from build123d import *

# Parameters (mm, degrees)
SKETCH1_R           = 2
SKETCH1_R_2         = 3.125
SKETCH1_R_3         = 1.7
BOSS_EXTRUDE1_DEPTH = 10
FILLET2_R           = 3
FILLET1_R           = 2
SKETCH1_4_R         = 3.125
CUT_EXTRUDE3_DEPTH  = 5.07
SKETCH1_7_R         = 1.7
CUT_EXTRUDE6_DEPTH  = 10
CUT_EXTRUDE5_DEPTH  = 3
SKETCH1_5_R         = 2
CUT_EXTRUDE4_DEPTH  = 2.48
SKETCH4_R           = 1.5
CUT_EXTRUDE7_DEPTH  = 10
SKETCH5_R           = 2.725
CUT_EXTRUDE8_DEPTH  = 2.8


with BuildPart() as part:
    # Sketch1 → Boss-Extrude1 (new body)
    with BuildSketch(Plane(origin=(0, 0, 0), x_dir=(1, 0, 0), z_dir=(0, 1, 0))):
        with BuildLine():
            ThreePointArc((-11.409245094, 8.977987014), (-9.849239736, 9.28), (-8.289234378, 8.977987014))
            ThreePointArc((-8.289234378, 8.977987014), (-5.835653376, 8.254222737), (-3.289234378, 8.01))
            Line((-3.289234378, 8.01), (38.12, 8.01))
            Line((38.12, 8.01), (38.12, -3.81))
            Line((38.12, -3.81), (28.478275237, -3.81))
            Line((28.478275237, -3.81), (26.178275237, 0))
            Line((26.178275237, 0), (-26.178275237, 0))
            Line((-26.178275237, 0), (-28.478275237, -3.81))
            Line((-28.478275237, -3.81), (-38.12, -3.81))
            Line((-38.12, -3.81), (-38.12, 8.01))
            Line((-38.12, 8.01), (-16.409245094, 8.01))
            ThreePointArc((-16.409245094, 8.01), (-13.862826096, 8.254222737), (-11.409245094, 8.977987014))
        make_face()
        with Locations((22, 4.005)):
            Circle(SKETCH1_R, mode=Mode.SUBTRACT)
        with Locations((-22, 4.005)):
            Circle(SKETCH1_R, mode=Mode.SUBTRACT)
        with Locations((-32.12, 1.98)):
            Circle(SKETCH1_R_2, mode=Mode.SUBTRACT)
        with Locations((32.12, 1.98)):
            Circle(SKETCH1_R_2, mode=Mode.SUBTRACT)
        with Locations((-9.849239736, 5.1)):
            Circle(SKETCH1_R_3, mode=Mode.SUBTRACT)
        with BuildLine():
            ThreePointArc((11.912105026, 2.53), (14.127105026, 4.745), (11.912105026, 6.96))
            Line((11.912105026, 6.96), (5.992105026, 6.96))
            ThreePointArc((5.992105026, 6.96), (3.777105026, 4.745), (5.992105026, 2.53))
            Line((5.992105026, 2.53), (11.912105026, 2.53))
        make_face(mode=Mode.SUBTRACT)
        with Locations((-22, 4.005)):
            Circle(SKETCH1_R)
        with Locations((-9.849239736, 5.1)):
            Circle(SKETCH1_R_3)
        with Locations((-32.12, 1.98)):
            Circle(SKETCH1_R_2)
        with BuildLine():
            Line((5.992105026, 2.53), (11.912105026, 2.53))
            ThreePointArc((11.912105026, 2.53), (14.127105026, 4.745), (11.912105026, 6.96))
            Line((11.912105026, 6.96), (5.992105026, 6.96))
            ThreePointArc((5.992105026, 6.96), (3.777105026, 4.745), (5.992105026, 2.53))
        make_face()
        with Locations((22, 4.005)):
            Circle(SKETCH1_R)
        with Locations((32.12, 1.98)):
            Circle(SKETCH1_R_2)
    extrude(amount=-BOSS_EXTRUDE1_DEPTH)

    # Fillet2
    fillet2_edges = [part.edges().sort_by_distance(p)[0] for p in [
        (28.478275237, -5, 3.81),
        (-28.478275237, -5, 3.81),
    ]]
    fillet(fillet2_edges, radius=FILLET2_R)

    # Fillet1
    fillet1_edges = [part.edges().sort_by_distance(p)[0] for p in [
        (26.178275237, -5, 0),
        (-26.178275237, -5, 0),
    ]]
    fillet(fillet1_edges, radius=FILLET1_R)

    # Sketch1_4 → Cut-Extrude3 (cut)
    with BuildSketch(Plane(origin=(0, 0, 0), x_dir=(1, 0, 0), z_dir=(0, 1, 0))):
        with Locations((32.12, 1.98)):
            Circle(SKETCH1_4_R)
        with Locations((-32.12, 1.98)):
            Circle(SKETCH1_4_R)
    extrude(amount=-CUT_EXTRUDE3_DEPTH, mode=Mode.SUBTRACT)

    # Sketch1_7 → Cut-Extrude6 (cut)
    with BuildSketch(Plane(origin=(0, 0, 0), x_dir=(1, 0, 0), z_dir=(0, 1, 0))):
        with Locations((-9.849239736, 5.1)):
            Circle(SKETCH1_7_R)
    extrude(amount=-CUT_EXTRUDE6_DEPTH, mode=Mode.SUBTRACT)

    # Sketch1_6 → Cut-Extrude5 (cut)
    with BuildSketch(Plane(origin=(0, 0, 0), x_dir=(1, 0, 0), z_dir=(0, 1, 0))):
        with BuildLine():
            Line((5.992105026, 2.53), (11.912105026, 2.53))
            ThreePointArc((11.912105026, 2.53), (14.127105026, 4.745), (11.912105026, 6.96))
            Line((11.912105026, 6.96), (5.992105026, 6.96))
            ThreePointArc((5.992105026, 6.96), (3.777105026, 4.745), (5.992105026, 2.53))
        make_face()
    extrude(amount=-CUT_EXTRUDE5_DEPTH, mode=Mode.SUBTRACT)

    # Sketch1_5 → Cut-Extrude4 (cut)
    with BuildSketch(Plane(origin=(0, 0, 0), x_dir=(1, 0, 0), z_dir=(0, 1, 0))):
        with Locations((-22, 4.005)):
            Circle(SKETCH1_5_R)
        with Locations((22, 4.005)):
            Circle(SKETCH1_5_R)
    extrude(amount=-CUT_EXTRUDE4_DEPTH, mode=Mode.SUBTRACT)

    # Sketch4 → Cut-Extrude7 (cut)
    with BuildSketch(Plane(origin=(0, 0, 0), x_dir=(1, 0, 0), z_dir=(0, 1, 0))):
        with Locations((-22, 4.005)):
            Circle(SKETCH4_R)
        with Locations((22, 4.005)):
            Circle(SKETCH4_R)
    extrude(amount=-CUT_EXTRUDE7_DEPTH, mode=Mode.SUBTRACT)

    # Sketch5 → Cut-Extrude8 (cut)
    with BuildSketch(Plane.XZ.offset(10)):
        with Locations((22, -4.005)):
            Circle(SKETCH5_R)
        with Locations((-22, -4.005)):
            Circle(SKETCH5_R)
    extrude(amount=-CUT_EXTRUDE8_DEPTH, mode=Mode.SUBTRACT)


solid = part.part
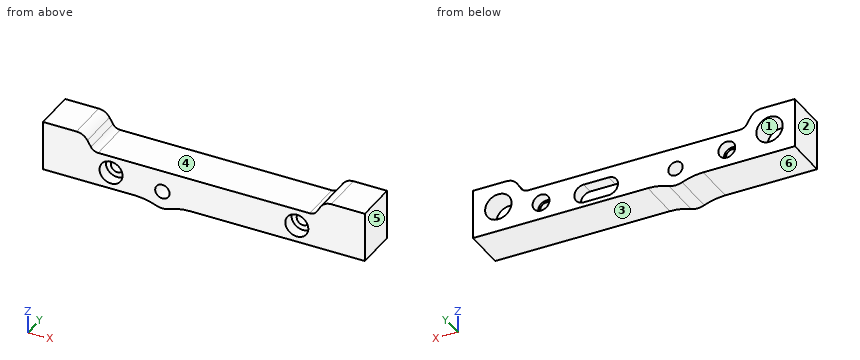
Design review of the part built by this model. Coordinates are the model's own, in mm. Face numbers are marked on the shaded views. A direction names the side the tool comes from. Give positions to 0.01 mm unless a question says otherwise; leave off trailing zeros. Loops run counter-clockwise (first coordinate to the right, second up) from the corner with the lowest first, then second, coordinate; pieces in that order, holes last. Notation, with made-up numbers: (2.5, 66.5) - (41.5, 66.5) arc R12 ccw to (41.5, 81.5) - close; hole circle Ø7 at (-17.5, 59). An arc over 180 degrees is marked (long way). Use CSV: the item, a comma, the result in double quotes. Start each with the question number.
1. Machinability: for the marked faces 1, 2 and 3, which of the approach directions +Z, -Z, +X, -X, +Y, -Y give a long, thin tool a straight path to every point of the face, cutting with its end or side? Answer none if there is none.
2. Wall thickness on L1, parallel to X at y = -2.95, z = -1.98 (3 decimals); L2, parallel to Z at x = 22, y = -4 (3 decimals); L3, parallel to X at y = -2.25, z = -5.5: over which ranges is each line inside the solid? List them lowest first.
3. Add section A-A (x = 22). State the section outline as (y, z) points (3 decimals).
4. Add section B-B (x = -32.12). State the section outline as (y, z) points (3 decimals), plus the area to 3 significant figures.
5. Draft analysis for pull direction X (two halves, no side actions). For the marked faces 4, 5 and 6, state which applies: released by +X, released by -X, zero draft, split by the parting line, or undercut.
6. Add section D-D (y = -0.75). Count the separate pieces of the cut face and the enclosed holes in it, plus the area to 3 significant figures.
7. Insertion check: P1, Ø2.5, axis at x = 8.5, y = -1.5, coming from the +Z side; P2, Ø3.5, axis at x = -22, z = -4.005, coming from the -Y side; P3, Ø3.5, axis at x = 22, z = -4.005, coming from the +Y side. Each pin has a flat end and moves straight along its axis. Give the tip position at first contact, or say it passes through.
8. Add section C-C (y = -6.5). State the section outline as (x, z) points (1 decimal).
Results found:
1,face 1,"+Y"
1,face 2,"+Z, -Z, -X, +Y, -Y"
1,face 3,"-Z, +X, +Y, -Y"
2,L1,"x = -38.12 to -35.245, -28.995 to 28.995, 35.245 to 38.12"
2,L2,"z = -8.01 to -5.505, -2.505 to 0"
2,L3,"x = -38.12 to -23.33, -20.67 to -11.5, -8.2 to 3.91, 13.99 to 20.67, 23.33 to 38.12"
3,outline,"(-10, -8.01) - (0, -8.01) - (0, -6.005) - (-2.48, -6.005) - (-2.48, -5.505) - (-7.2, -5.505) - (-7.2, -6.73) - (-10, -6.73) - close; (-10, -1.28) - (-7.2, -1.28) - (-7.2, -2.505) - (-2.48, -2.505) - (-2.48, -2.005) - (0, -2.005) - (0, 0) - (-10, 0) - close"
4,outline,"(-10, -8.01) - (0, -8.01) - (0, -5.105) - (-5.07, -5.105) - (-5.07, 1.145) - (0, 1.145) - (0, 3.81) - (-10, 3.81) - close"
4,area,"86.5 mm²"
5,face 4,"undercut"
5,face 5,"released by +X"
5,face 6,"zero draft"
6,separate pieces,"1"
6,enclosed holes,"6"
6,area,"562 mm²"
7,P1,"stops at z = 0"
7,P2,"stops at y = -7.2"
7,P3,"stops at y = -2.48"
8,outline,"(-38.1, -8) - (-16.4, -8) arc R13.4 cw to (-11.4, -9) arc R4.2 ccw to (-8.3, -9) arc R13.4 cw to (-3.3, -8) - (38.1, -8) - (38.1, 3.8) - (30.2, 3.8) arc R3 ccw to (27.6, 2.4) - (26.8, 1) arc R2 cw to (25, 0) - (-25, 0) arc R2 cw to (-26.8, 1) - (-27.6, 2.4) arc R3 ccw to (-30.2, 3.8) - (-38.1, 3.8) - close; hole circle Ø3 at (-22, -4); hole circle Ø3.4 at (-9.8, -5.1); hole circle Ø3 at (22, -4)"
